Verification items for the finished model (mm, model axes). Face numbers are marked on the shaded views. A direction names the side the tool comes from. Coordinates: 2 decimals unless noted, no trailing zeros. Loops run counter-clockwise (first coordinate to the right, second up) from the corner with the lowest first, then second, coordinate; pieces in that order, holes last. Notation, with made-up numbers: (-7.5, 10.5) -> (42.5, 10.5) arc R30 ccw to (42.5, 43.5) -> close; hole circle Ø1 at (15.5, 69). An arc over 180 degrees is marked (long way). Write item = value, one per line.
```python
from build123d import *

# Parameters (mm, degrees)
SKETCH1_R           = 5
BOSS_EXTRUDE1_DEPTH = 20
SKETCH2_R           = 8.6
BOSS_EXTRUDE2_DEPTH = 5
FILLET1_SIZE        = 2.5
FILLET1_SIZE_2      = 4
CUT_EXTRUDE1_DEPTH  = 4
FILLET2_R           = 0.5
CHAMFER1_SIZE       = 0.5


with BuildPart() as part:
    # Sketch1 → Boss-Extrude1 (new body)
    with BuildSketch(Plane(origin=(0, 0, 0), x_dir=(1, 0, 0), z_dir=(0, 1, 0))):
        with Locations(Location((0, 0, 0), (0, 0, 270))):
            Circle(SKETCH1_R)
    extrude(amount=BOSS_EXTRUDE1_DEPTH)

    # Sketch2 → Boss-Extrude2 (add)
    with BuildSketch(Plane(origin=(0, 20, 0), x_dir=(1, 0, 0), z_dir=(0, 1, 0))):
        with Locations(Location((0, 0, 0), (0, 0, 270))):
            Circle(SKETCH2_R)
    extrude(amount=BOSS_EXTRUDE2_DEPTH)

    # Fillet1
    # an asymmetric fillet: 4, 2.5 mm, written as the material it takes off along each edge
    with BuildSketch(Plane(origin=(0, 25, 0), x_dir=(0, 0, 1), z_dir=(-1, 0, 0))) as fillet1_piece_1:
        with BuildLine():
            Bezier((8.6, -FILLET1_SIZE), (8.6, 0), (8.6 - FILLET1_SIZE_2, 0), weights=[1, 0.707106781, 1])
            Line((8.6 - FILLET1_SIZE_2, 0), (8.6, 0))
            Line((8.6, 0), (8.6, -FILLET1_SIZE))
        make_face()
    revolve(axis=Axis((0, 25, 0), (0, 1, 0)), mode=Mode.SUBTRACT)

    # Sketch3 → Cut-Extrude1 (cut)
    with BuildSketch(Plane(origin=(0, 25, 0), x_dir=(1, 0, 0), z_dir=(0, 1, 0))):
        Polygon((2.501014418, -2.520402127), (3.433239479, 0.905740958), (0.93222506, 3.426143085), (-2.501014418, 2.520402127), (-3.433239479, -0.905740958), (-0.93222506, -3.426143085), align=None)
    extrude(amount=-CUT_EXTRUDE1_DEPTH, mode=Mode.SUBTRACT)

    # Fillet2
    fillet2_edges = [part.edges().sort_by_distance(p)[0] for p in [
        (0, 20, -8.6),
    ]]
    fillet(fillet2_edges, radius=FILLET2_R)

    # Chamfer1
    chamfer1_edges = [part.edges().sort_by_distance(p)[0] for p in [
        (0, 0, -5),
    ]]
    chamfer(chamfer1_edges, length=CHAMFER1_SIZE)


solid = part.part
```
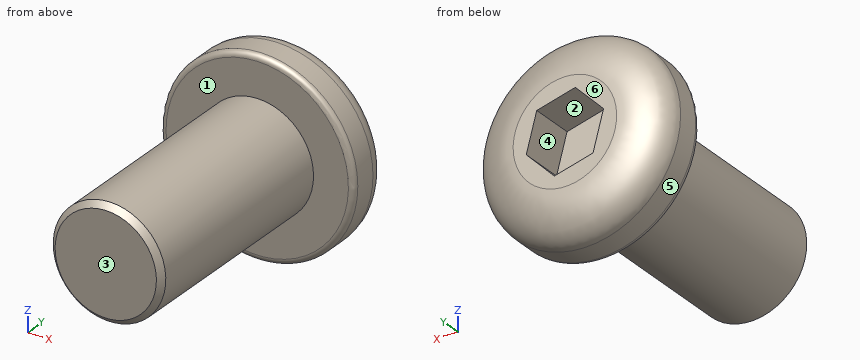
1) Release check for a two-part mould opening along Z. For the marked faces 4, 5 and 6 record: pulls with the +Z half, pulls with the -Z half, needs draft (parallel to the pull), parting line crosses it, or undercut.
Ans:
face_4 = undercut
face_5 = parting line crosses it
face_6 = needs draft
2) Sectioned sample at B-B, the plane y = 13. Record the cut outline in (x, z), plus the area to 3 significant figures.
Ans:
outline = circle Ø10 at (0, 0)
area = 78.5 mm2
3) Depth check by flat-ended pin: pin 1 Ø8 at (y, z) = (5.5, -0.5) entering from -X; pin 2 Ø3 at (x, z) = (-6.5, -1.5) entering from +Y; pin 3 Ø4 at (x, y) = (5.5, 11) entering from +Z. Enter the tip coordinate at first touch or a pass-through.
Ans:
pin_1 = -5
pin_2 = 24.97
pin_3 = 3.57
4) Sectioned sample at A-A, the plane y = 21.75. Record the cut outline in (x, z), plus the area to 3 significant figures.
Ans:
outline = circle Ø17.2 at (0, 0); hole (-3.43, 0.91) -> (-2.5, -2.52) -> (0.93, -3.43) -> (3.43, -0.91) -> (2.5, 2.52) -> (-0.93, 3.43) -> close
area = 200 mm2
5) Material ranges on line 1 (Z direction, x = -3.75, y = 5.5); line 2 (Z direction, x = -2, y = 7.75); line 3 (X direction, y = 4.5, z = 3), recorded low to high.
Ans:
line_1 = -3.31 to 3.31
line_2 = -4.58 to 4.58
line_3 = -4 to 4
6) Tool access check on the marked faces 1, 2 and 3. Record the directions out of +Z, -Z, +X, -X, +Y, -Y that give a thin tool (end or side, any length) a straight path to the whole face; none if there is none.
Ans:
face_1 = -Y
face_2 = +Y
face_3 = +Z, -Z, +X, -X, -Y
